Model file for the job. Use its own axes, mm. A direction names the side the tool comes from. Round coordinates to 2 decimals unless told otherwise and drop trailing zeros. Loops run counter-clockwise (first coordinate to the right, second up) from the corner with the lowest first, then second, coordinate; pieces in that order, holes last. Notation, with made-up numbers: M 21.25,35.5 L 37.25,35.5 A26 cw 37.25,69.5 Z; hole C -29,88.25 d4. An arc over 180 degrees is marked long. Use a Markdown table: item, result. Add a question column.
Q1. Probe line 1 (X direction, y = -4.75, z = 3); line 2 (X direction, y = 0.25, z = 0.7); line 3 (X direction, y = -0.75, z = 3.55). List the from-to ranges inside material, lowest first. Write a range as from..to.
Q2. Mould opens along Y. For faces 3 (the face through (9.1, 0.07, 2.71)), 4 (the face through (9.43, 9.4, 2.79)), 5 (the face through (5.7, 0.1, 5.5)) say: +Y half, -Y half, draft (parallel to the pull), parting line (faces both ways), or undercut.
Q3. Tool access for faces 1 (the face through (-4, 0, 4)), 2 (the face through (-10, 0, 3)): list every direction of +Z, -Z, +X, -X, +Y, -Y with a clear straight run to the whole face (end or side of a thin tool).
Q4. Cut at C-C (y = 0). Give the cut face in (x, z).
Q5. Pin check, flat tips, straight feed: pin 1 (2.5 mm diameter, centred on x = 7.5, y = 0, fed in from -Z); pin 2 (2.5 mm diameter, centred on x = 0, y = -1.5, fed in from +Z); pin 3 (3 mm diameter, centred on x = -2.5, y = 1.5, fed in from -Z). Stop position of each tip, or through.
Q6. Cut at D-D (z = 0.55). Give the cut face in (x, y), plus the area to 3 significant figures.
Q7. Cut at A-A (x = 7.5). Give the cut face in (y, z).
Q8. Cut at B-B (z = 3.2). Give the cut face in (x, y), plus the area to 3 significant figures.
from build123d import *

# Parameters (mm, degrees)
SKETCH1_W           = 20
SKETCH1_H           = 20
BOSS_EXTRUDE1_DEPTH = 5.5
SKETCH2_W           = 8
SKETCH2_H           = 3.5
CUT_EXTRUDE1_DEPTH  = 24.027157879
HOLEWZD1_D          = 3.2
FILLET1_R           = 2


with BuildPart() as part:
    # Sketch1 → Boss-Extrude1 (new body)
    with BuildSketch(Plane(origin=(0, 0, 0), x_dir=(-1, 0, 0), z_dir=(0, 0, -1))):
        Rectangle(SKETCH1_W, SKETCH1_H)
    extrude(amount=-BOSS_EXTRUDE1_DEPTH)

    # Sketch2 → Cut-Extrude1 (cut, through all)
    with BuildSketch(Plane(origin=(0, 10, 0), x_dir=(-1, 0, 0), z_dir=(0, 1, 0))):
        with Locations((0, 3.75)):
            Rectangle(SKETCH2_W, SKETCH2_H)
    extrude(amount=-CUT_EXTRUDE1_DEPTH, mode=Mode.SUBTRACT)

    # HoleWzd1 (through all)
    with Locations(Plane.XY.offset(5.5)):
        with Locations((7.5, 0), (-7.5, 0)):
            Hole(HOLEWZD1_D / 2)

    # Fillet1
    fillet1_edges = [part.edges().sort_by_distance(p)[0] for p in [
        (-10, -10, 2.75),
        (10, -10, 2.75),
        (10, 10, 2.75),
        (-10, 10, 2.75),
    ]]
    fillet(fillet1_edges, radius=FILLET1_R)


solid = part.part
Checked values:
| question | item | result |
|---|---|---|
| 1 | line 1 | x = -10..-4, 4..10 |
| 1 | line 2 | x = -10..-9.08, -5.92..5.92, 9.08..10 |
| 1 | line 3 | x = -10..-8.91, -6.09..-4, 4..6.09, 8.91..10 |
| 2 | face 3 | undercut |
| 2 | face 4 | +Y half |
| 2 | face 5 | draft |
| 3 | face 1 | +Z, +Y, -Y |
| 3 | face 2 | +Z, -Z, -X, +Y, -Y |
| 4 | outline | M -10,0 L -9.1,0 L -9.1,5.5 L -10,5.5 Z; M -5.9,0 L 5.9,0 L 5.9,5.5 L 4,5.5 L 4,2 L -4,2 L -4,5.5 L -5.9,5.5 Z; M 9.1,0 L 10,0 L 10,5.5 L 9.1,5.5 Z |
| 5 | pin 1 | passes through |
| 5 | pin 2 | stops at z = 2 |
| 5 | pin 3 | stops at z = 0 |
| 6 | outline | M -10,-8 A2 ccw -8,-10 L 8,-10 A2 ccw 10,-8 L 10,8 A2 ccw 8,10 L -8,10 A2 ccw -10,8 Z; hole C -7.5,0 d3.2; hole C 7.5,0 d3.2 |
| 6 | area | 380 mm^2 |
| 7 | outline | M -10,0 L -1.6,0 L -1.6,5.5 L -10,5.5 Z; M 1.6,0 L 10,0 L 10,5.5 L 1.6,5.5 Z |
| 8 | outline | M -10,-8 A2 ccw -8,-10 L -4,-10 L -4,10 L -8,10 A2 ccw -10,8 Z; M 4,-10 L 8,-10 A2 ccw 10,-8 L 10,8 A2 ccw 8,10 L 4,10 Z; hole C -7.5,0 d3.2; hole C 7.5,0 d3.2 |
| 8 | area | 220 mm^2 |
